The drawing under review shows one solid part. Ordinate dimensions are in mm from its lowest x, y, z. Coordinates: 2 decimals unless noted, no trailing zeros. Order: outer loops, then holes, each group sorted by start corner. A loop starts at its lowest first (then second) coordinate and runs counter-clockwise, first axis right, second up. Notation, with made-up numbers: (38.25, 78.25) -> (59.25, 78.25) arc R23 ccw to (59.25, 112.25) -> close; hole circle Ø4 at (5, 68.25). An arc over 180 degrees is marked (long way). Put each result on its own line as item: value.
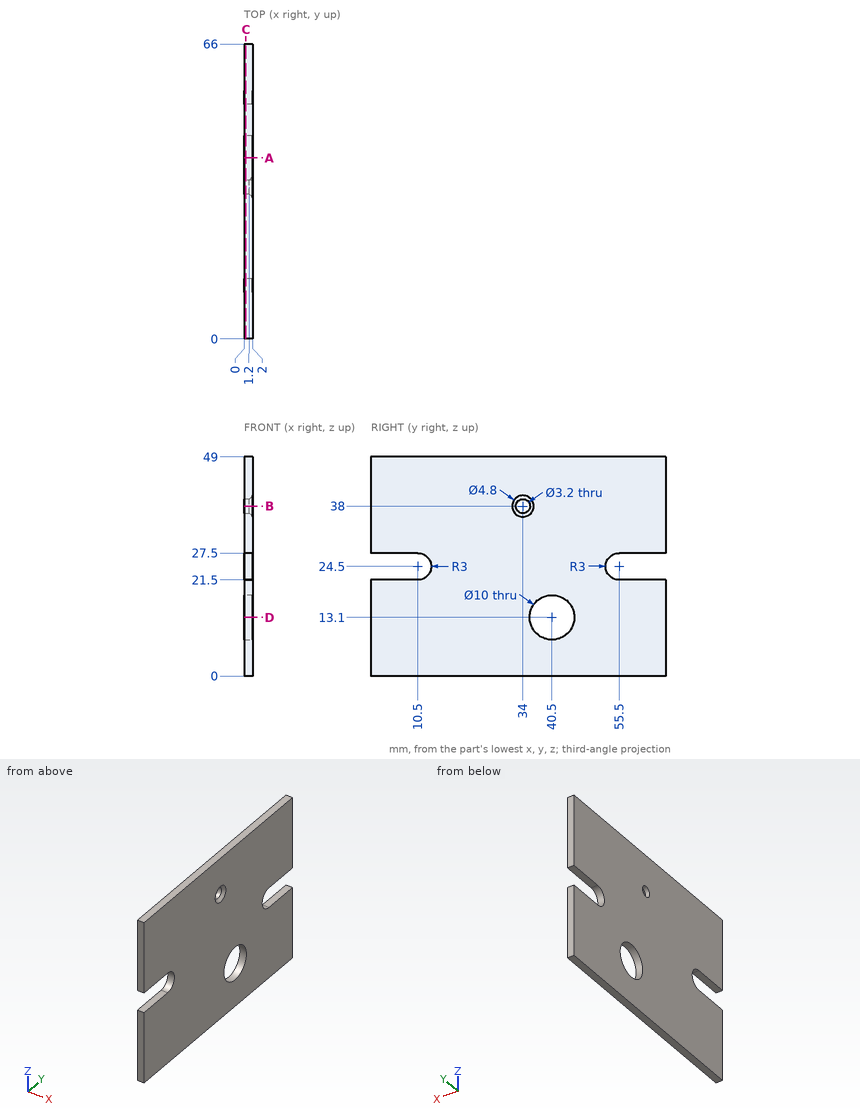
Item 1: Consider section D-D on z = 13.1. Write out the cut boundary in (x, y).
Answers below:
outline: (0, 0) -> (2, 0) -> (2, 35.5) -> (0, 35.5) -> close; (0, 45.5) -> (2, 45.5) -> (2, 66) -> (0, 66) -> close
Item 2: Consider section B-B on z = 38. Write out the cut boundary in (x, y).
Answers below:
outline: (0, 0) -> (2, 0) -> (2, 31.6) -> (1.2, 32.4) -> (0, 32.4) -> close; (0, 35.6) -> (1.2, 35.6) -> (2, 36.4) -> (2, 66) -> (0, 66) -> close
Item 3: Consider section A-A on y = 40.5. Write out the cut boundary in (x, z).
Answers below:
outline: (0, 0) -> (2, 0) -> (2, 8.1) -> (0, 8.1) -> close; (0, 18.1) -> (2, 18.1) -> (2, 49) -> (0, 49) -> close
Item 4: For line 1 (Z direction, x = 0.65, y = 40.5); line 2 (Z direction, x = 0.7, y = 34); line 3 (Y direction, x = 0.9, z = 38), list the stretches that pass through material, from the lowest coordinate up. Write a range as from..to.
Answers below:
line 1: 0..8.1, 18.1..49
line 2: 0..36.4, 39.6..49
line 3: 0..32.4, 35.6..66
Item 5: Consider section C-C on x = 0.4. Write out the cut boundary in (y, z), and give its area (3 significant figures).
Answers below:
outline: (0, 0) -> (66, 0) -> (66, 21.5) -> (55.5, 21.5) arc R3 cw to (55.5, 27.5) -> (66, 27.5) -> (66, 49) -> (0, 49) -> (0, 27.5) -> (10.5, 27.5) arc R3 cw to (10.5, 21.5) -> (0, 21.5) -> close; hole circle Ø3.2 at (34, 38); hole circle Ø10 at (40.5, 13.1)
area: 2,990 mm^2
